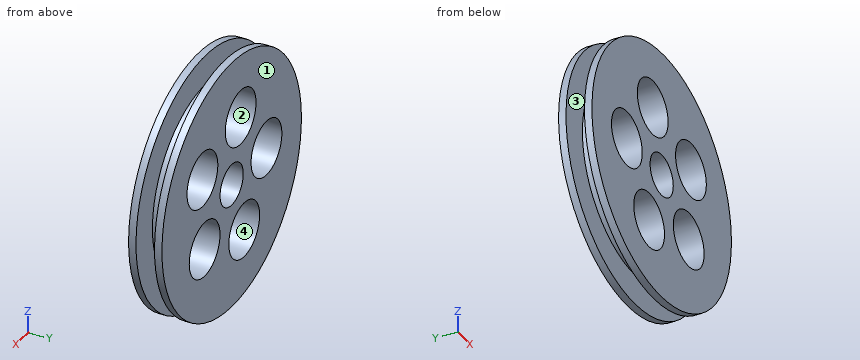
from build123d import *

# Parameters (mm, degrees)
SKETCH1_W          = 22
SKETCH1_H          = 5
SKETCH1_W_2        = 30
SKETCH1_H_2        = 2
SKETCH3_R          = 5.653749864
SKETCH3_R_2        = 7.5
CUT_EXTRUDE1_DEPTH = 10


with BuildPart() as part:
    # Sketch1 → Revolve4 (revolve)
    with BuildSketch(Plane(origin=(0, 0, 0), x_dir=(0, 0, -1), z_dir=(1, 0, 0))):
        Polygon((0, 7), (0, 5), (22, 5), (30, 5), (30, 7), align=None)
        with Locations((11, 2.5)):
            Rectangle(SKETCH1_W, SKETCH1_H)
        with Locations((15, -1)):
            Rectangle(SKETCH1_W_2, SKETCH1_H_2)
    revolve(axis=Axis((0, 2.5, 4), (0, 1, 0)))

    # Sketch3 → Cut-Extrude1 (cut)
    with BuildSketch(Plane(origin=(0, 7, 0), x_dir=(1, 0, 0), z_dir=(0, 1, 0))):
        with Locations((0, -4)):
            Circle(SKETCH3_R)
        with Locations((-16.975218646, -4.917579386)):
            Circle(SKETCH3_R_2)
        with Locations((-6.118300899, 11.860844685)):
            Circle(SKETCH3_R_2)
        with Locations((13.193900737, 6.720120492)):
            Circle(SKETCH3_R_2)
        with Locations((14.272579999, -13.235445857)):
            Circle(SKETCH3_R_2)
        with Locations((-4.37296119, -20.427939933)):
            Circle(SKETCH3_R_2)
    extrude(amount=-CUT_EXTRUDE1_DEPTH, mode=Mode.SUBTRACT)


solid = part.part
Can you work these out from the model? Positions are in its coordinate system, mm. Face numbers are marked on the shaded views. A direction names the side the tool comes from. Coordinates: 2 decimals unless noted, no trailing zeros. Loops run counter-clockwise (first coordinate to the right, second up) from the corner with the lowest first, then second, coordinate; pieces in that order, holes last. Notation, with made-up numbers: (-16.5, 11) - (-11.5, 11) arc R20 cw to (-11.5, 20) - close; hole circle Ø8 at (-33, -1). An arc over 180 degrees is marked (long way). Answer as a JSON object with one key per item and string values. Group by question number.
Item 1: If we section it at A-A (z = -25): List the corners of the cut face in (x, y) for me.
Item 2: If we mould it in two halves opening along Z, with no side actions, what happens to the marked faces 1 and 2? For each: released by +Z, released by -Z, zero draft, split by the parting line, or undercut.
Item 3: If we section it at C-C (z = 4): List the corners of the cut face in (x, y) for me, plus the area to 3 significant figures.
Item 4: For pin 1 (1 mm diameter, centred on x = 3.5, y = 1.5, fed in from +Z); pin 2 (9 mm diameter, centred on x = 14.27, z = 13.24, fed in from +Y); pin 3 (1 mm diameter, centred on y = 1, z = 18.5, fed in from +X), each with a flat end and sliding along its axis, tell me the tip position at first contact or that it passes through.
Item 5: If we section it at D-D (x = 13.5): List the corners of the cut face in (y, z) for me, plus the area to 3 significant figures.
Item 6: If I drill on L1, parallel to Z at x = -4.5, y = 3.25; L2, parallel to Z at x = 11, y = -1; L3, parallel to Y at x = -30, z = 5, over which ranges is the centre line in solid material (lowest first)? Write a range as from..to.
Item 7: On a 3-axis mill with a long thin cutter (end or side, diameter ignored), from which of +Z, -Z, +X, -X, +Y, -Y can I reach the whole of each face in a straight line? I mean the marked faces 3 and 4. Say none if no direction works.
Item 8: If we section it at B-B (x = 0): List the corners of the cut face in (y, z) for me.
Returned:
{
 "1": {"outline": "(-17.75, -2) - (17.75, -2) - (17.75, 0) - (-17.75, 0) - close; (-17.75, 5) - (17.75, 5) - (17.75, 7) - (-17.75, 7) - close"},
 "2": {"face 1": "zero draft", "face 2": "undercut"},
 "3": {"outline": "(-34, -2) - (-24.42, -2) - (-24.42, 7) - (-34, 7) - (-34, 5) - (-26, 5) - (-26, 0) - (-34, 0) - close; (-9.53, -2) - (-5.65, -2) - (-5.65, 7) - (-9.53, 7) - close; (5.65, -2) - (34, -2) - (34, 0) - (26, 0) - (26, 5) - (34, 5) - (34, 7) - (5.65, 7) - close", "area": "296 mm²"},
 "4": {"pin 1": "stops at z = 29.83", "pin 2": "passes through", "pin 3": "stops at x = 21.91"},
 "5": {"outline": "(-2, -27.2) - (0, -27.2) - (0, -18.22) - (5, -18.22) - (5, -27.2) - (7, -27.2) - (7, -14.21) - (-2, -14.21) - close; (-2, 0.77) - (7, 0.77) - (7, 5.78) - (-2, 5.78) - close; (-2, 20.7) - (7, 20.7) - (7, 35.2) - (5, 35.2) - (5, 26.22) - (0, 26.22) - (0, 35.2) - (-2, 35.2) - close", "area": "203 mm²"},
 "6": {"L1": "z = -21.61..-19.18, -4.54..0.58, 7.42..12.93, 27.93..29.61", "L2": "z = -28.17..-13.89, 0.45..6.49, 19.98..36.17", "L3": "y = -2..0, 5..7"},
 "7": {"face 3": "none", "face 4": "+Y, -Y"},
 "8": {"outline": "(-2, -30) - (0, -30) - (0, -22) - (5, -22) - (5, -30) - (7, -30) - (7, -16.2) - (-2, -16.2) - close; (-2, -7.52) - (7, -7.52) - (7, -1.65) - (-2, -1.65) - close; (-2, 9.65) - (7, 9.65) - (7, 14.33) - (-2, 14.33) - close; (-2, 26.52) - (7, 26.52) - (7, 38) - (5, 38) - (5, 30) - (0, 30) - (0, 38) - (-2, 38) - close"}
}
